The listing builds one solid part. Answer for the finished solid, in the listing's coordinates (mm). Face numbers are marked on the shaded views. A direction names the side the tool comes from. Coordinates: 2 decimals unless noted, no trailing zeros. Order: outer loops, then holes, each group sorted by start corner. A loop starts at its lowest first (then second) coordinate and runs counter-clockwise, first axis right, second up. Notation, with made-up numbers: (79, -39.75) - (107, -39.75) arc R13 ccw to (107, -29.75) - close; hole circle Ø8 at (24.5, 39). An arc over 180 degrees is marked (long way). One line per item, written item: value. Start each with the question number.
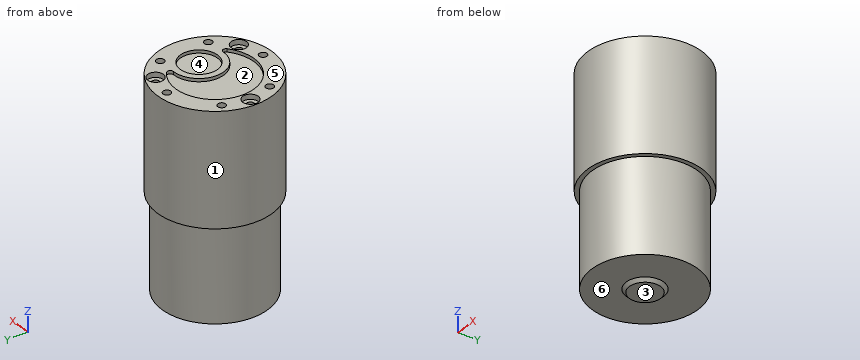
```python
from build123d import *

# Parameters (mm, degrees)
TALADRO_ROSCADO_M3X0_52_D                            = 2.5
TALADRO_ROSCADO_M3X0_52_DEPTH                        = 8.5
TALADRO_ROSCADO_M3X0_52_TIP                          = 0.751075774
REFRENTADO_PARA_TORNILLO_CON_CABEZA_TRON_D           = 2.4
REFRENTADO_PARA_TORNILLO_CON_CABEZA_TRON_DEPTH       = 5
REFRENTADO_PARA_TORNILLO_CON_CABEZA_TRON_CBORE_D     = 5
REFRENTADO_PARA_TORNILLO_CON_CABEZA_TRON_CBORE_DEPTH = 1.6
REFRENTADO_PARA_TORNILLO_CON_CABEZA_TRON_TIP         = 0.721032743
CROQUIS8_R                                           = 6
CORTAR_EXTRUIR2_DEPTH                                = 1


with BuildPart() as part:
    # Croquis1 → Revolución1 (revolve)
    with BuildSketch(Plane(origin=(0, 0, 0), x_dir=(0, 0, -1), z_dir=(1, 0, 0)), mode=Mode.PRIVATE) as revoluci_n1_sk:
        Polygon((-33.5, 0), (33.5, 0), (33.5, 5), (32.5, 6), (32.5, 17), (2.5, 17), (2.5, 18.4), (-33.5, 18.4), align=None)
    revolve(revoluci_n1_sk.sketch.rotate(Axis((0, 0, 33.5), (0, 0, -1)), 90), axis=Axis((0, 0, 33.5), (0, 0, -1)))

    # Taladro roscado M3x0.52
    with Locations(Plane.XY.offset(33.5)):
        with Locations((0, 15.5), (0, -15.5), (13.423393759, -7.75), (13.423393759, 7.75), (-13.423393759, 7.75), (-13.423393759, -7.75)):
            Hole(TALADRO_ROSCADO_M3X0_52_D / 2, depth=TALADRO_ROSCADO_M3X0_52_DEPTH)
            with Locations((0, 0, -(TALADRO_ROSCADO_M3X0_52_DEPTH + TALADRO_ROSCADO_M3X0_52_TIP / 2))):  # 118° drill point
                Cone(0, TALADRO_ROSCADO_M3X0_52_D / 2, TALADRO_ROSCADO_M3X0_52_TIP, mode=Mode.SUBTRACT)

    # Refrentado para tornillo con cabeza troncocónica de M21
    with Locations(Plane.XY.offset(33.5)):
        with Locations((-15.5, 0), (7.75, 13.423393759), (7.75, -13.423393759)):
            CounterBoreHole(REFRENTADO_PARA_TORNILLO_CON_CABEZA_TRON_D / 2, REFRENTADO_PARA_TORNILLO_CON_CABEZA_TRON_CBORE_D / 2, REFRENTADO_PARA_TORNILLO_CON_CABEZA_TRON_CBORE_DEPTH, depth=REFRENTADO_PARA_TORNILLO_CON_CABEZA_TRON_DEPTH)
            with Locations((0, 0, -(REFRENTADO_PARA_TORNILLO_CON_CABEZA_TRON_DEPTH + REFRENTADO_PARA_TORNILLO_CON_CABEZA_TRON_TIP / 2))):  # 118° drill point
                Cone(0, REFRENTADO_PARA_TORNILLO_CON_CABEZA_TRON_D / 2, REFRENTADO_PARA_TORNILLO_CON_CABEZA_TRON_TIP, mode=Mode.SUBTRACT)

    # Croquis8 → Cortar-Extruir2 (cut)
    with BuildSketch(Plane.XY.offset(33.5)):
        with Locations((7, 0)):
            Circle(CROQUIS8_R)
        with BuildLine():
            ThreePointArc((7.957241379, 9.769458001), (-12.6, 0), (7.957241379, -9.769458001))
            ThreePointArc((7.957241379, -9.769458001), (8.261660496, -8.641961193), (7.28952381, -7.994759281))
            ThreePointArc((7.28952381, -7.994759281), (-1, 0), (7.28952381, 7.994759281))
            ThreePointArc((7.28952381, 7.994759281), (8.261660496, 8.641961193), (7.957241379, 9.769458001))
        make_face()
    extrude(amount=-CORTAR_EXTRUIR2_DEPTH, mode=Mode.SUBTRACT)


solid = part.part
```
(1) Consider probe 1 along Y at (x, z) = (0, 31); probe 2 along X at (y, z) = (-7.75, 28.25); probe 3 along Z at (x, y) = (-7, 14.5). Determine where each line is inside the solid, lowest interval first.
(2) Flat-ended cylindrical pins translate along their axes: pin 1 Ø1.5 at (x, y) = (7.5, 14) entering from +Z; pin 2 Ø1.5 at (x, z) = (-0.5, 12) entering from -Y; pin 3 Ø12 at (y, z) = (-8, -0.5) entering from +X. Find the tip coordinate at first contact, or state that the pin passes through.
(3) The part is cut by section A-A on z = -4. Determine the outline of the cut face in (x, y).
(4) For the marked faces 5 and 6, determine the directions among +Z, -Z, +X, -X, +Y, -Y from which every point of the face is accessible in a straight line to the end or side of a thin tool.
(5) For a pull along Y with two mould halves and no side action, classify the marked faces 1, 2, 3 and 4 as pulls with the +Y half, pulls with the -Y half, needs draft (parallel to the pull), parting line crosses it, or undercut.
Completed:
1. probe 1: y = -18.4 to -16.75, -14.25 to 14.25, 16.75 to 18.4
1. probe 2: x = -16.69 to -14.67, -12.17 to 12.17, 14.67 to 16.69
1. probe 3: z = -32.5 to 33.5
2. pin 1: stops at z = 31.9
2. pin 2: stops at y = -18.4
2. pin 3: stops at x = 18.29
3. outline: circle Ø34 at (0, 0)
4. face 5: +Z, +X, -X, +Y, -Y
4. face 6: -Z
5. face 1: parting line crosses it
5. face 2: undercut
5. face 3: needs draft
5. face 4: undercut
